Drawing for the job (mm, zero at the part's lowest x, y, z). A direction names the side the tool comes from. Round coordinates to 2 decimals unless told otherwise and drop trailing zeros. Write each loop counter-clockwise with the first axis right and the second up, starting at its lowest first coordinate (ties: lowest second). Pieces come first, ordered by that corner, then holes. Notation, with made-up numbers: M 47.25,2.5 L 59.25,2.5 A32 ccw 59.25,36.5 Z; hole C -27,18.25 d8. An arc over 180 degrees is marked long. Use a Markdown table: item, result. Add a question column.
1) Two-plate mould, pull along Z, no slides. Class the marked faces 1, 2 and 3: released by +Z, released by -Z, zero draft, split by the parting line, or undercut.
2) Drop flat-ended pins along their axis: P1, Ø1, axis at x = 38.5, z = 13.5, coming from the -Y side; P2, Ø2.5, axis at x = 45, z = 42.5, coming from the -Y side; P3, Ø16, axis at x = 32.5, y = 36.5, coming from the -Z side. Give the stop position or say it passes through.
3) Wall check: probe 1 along Y at (x, z) = (49, 30) (3 decimals); probe 2 along Z at (x, y) = (42.5, 25); probe 3 along Y at (x, z) = (43.6, 30) (1 decimal). Give the ranges that are in metal, low to high.
4) Slice it at D-D on y = 70.5. Write the cut outline in (x, z).
5) Slice it at C-C on x = 33. Write the cut outline in (y, z).
6) Slice it at A-A on y = 21.56. Write the cut outline in (x, z), plus the area to 3 significant figures.
7) Slice it at B-B on z = 30. Give the number of separate pieces and of enclosed holes in the cut face, plus the area to 3 significant figures.
8) Which spindle directions (+Z, -Z, +X, -X, +Y, -Y) get a long thin tool onto all of the face, cutting with end or side? Do the marked faces 4, 5 and 6. Say none if no direction does.
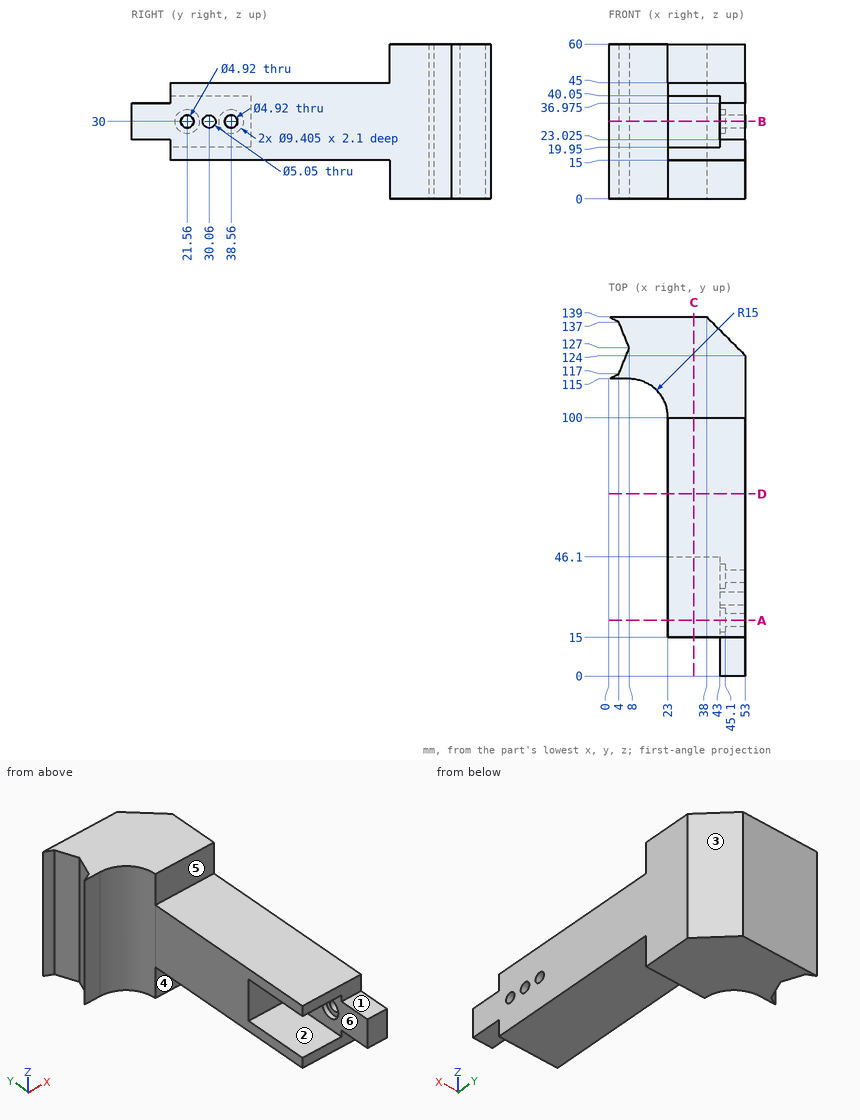
Entries:
| question | item | result |
|---|---|---|
| 1 | face 1 | released by +Z |
| 1 | face 2 | undercut |
| 1 | face 3 | zero draft |
| 2 | P1 | stops at y = 100 |
| 2 | P2 | stops at y = 15 |
| 2 | P3 | stops at z = 15 |
| 3 | probe 1 | y = 0 to 19.1, 24.02 to 27.535, 32.585 to 36.1, 41.02 to 128 |
| 3 | probe 2 | z = 15 to 19.95, 40.05 to 45 |
| 3 | probe 3 | y = 0 to 16.9, 26.3 to 27.5, 32.6 to 33.9, 43.3 to 133.4 |
| 4 | outline | M 23,15 L 53,15 L 53,45 L 23,45 Z |
| 5 | outline | M 15,15 L 100,15 L 100,0 L 139,0 L 139,60 L 100,60 L 100,45 L 15,45 L 15,40.05 L 46.1,40.05 L 46.1,19.95 L 15,19.95 Z |
| 6 | outline | M 23,15 L 53,15 L 53,27.54 L 45.1,27.54 L 45.1,25.3 L 43,25.3 L 43,19.95 L 23,19.95 Z; M 23,40.05 L 43,40.05 L 43,34.7 L 45.1,34.7 L 45.1,32.46 L 53,32.46 L 53,45 L 23,45 Z |
| 6 | area | 439 mm^2 |
| 7 | separate pieces | 4 |
| 7 | enclosed holes | 0 |
| 7 | area | 3,440 mm^2 |
| 8 | face 4 | -Z, +X, -X, -Y |
| 8 | face 5 | +Z, +X, -X, -Y |
| 8 | face 6 | -X, -Y |
